Check sheet for the drawn part. Datum: minimum x, y, z corner. Units: mm. Round coordinates to 2 decimals unless told otherwise and drop trailing zeros. Write each loop counter-clockwise with the first axis right and the second up, starting at its lowest first coordinate (ties: lowest second). Pieces come first, ordered by that corner, then holes.
Item 1: Material ranges on line 1 (X direction, y = 33.5, z = 2.8); line 2 (Y direction, x = 46, z = 1.1), recorded low to high.
Item 2: Cross-section at B-B on z = 1.7. Enter the section's corners in (x, y).
Item 3: Cross-section at A-A on y = 2. Enter the section's corners in (x, z).
Item 4: Cross-section at C-C on x = 42.5. Enter the section's corners in (y, z).
Item 5: Go/stop test with flat-tipped pins: pin 1 Ø0.9 at (y, z) = (1.5, 2) entering from -X; pin 2 Ø1.5 at (y, z) = (34.5, 2) entering from +X. Record where each tip stops, or that it passes through.
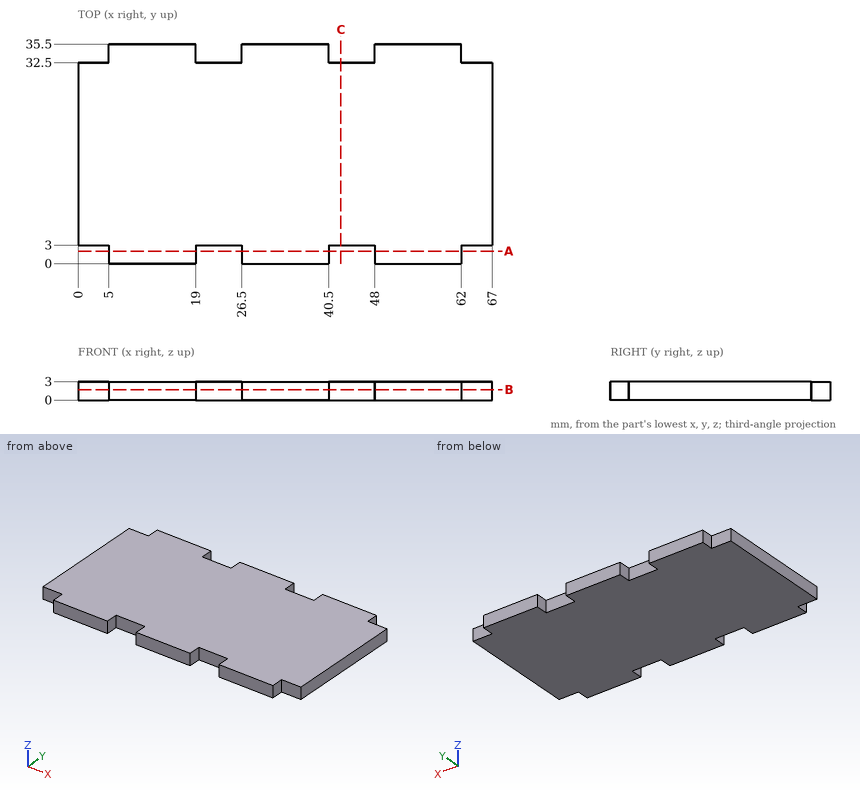
Response values:
1. line 1: x = 5 to 19, 26.5 to 40.5, 48 to 62
1. line 2: y = 3 to 32.5
2. outline: (0, 3) - (5, 3) - (5, 0) - (19, 0) - (19, 3) - (26.5, 3) - (26.5, 0) - (40.5, 0) - (40.5, 3) - (48, 3) - (48, 0) - (62, 0) - (62, 3) - (67, 3) - (67, 32.5) - (62, 32.5) - (62, 35.5) - (48, 35.5) - (48, 32.5) - (40.5, 32.5) - (40.5, 35.5) - (26.5, 35.5) - (26.5, 32.5) - (19, 32.5) - (19, 35.5) - (5, 35.5) - (5, 32.5) - (0, 32.5) - close
3. outline: (5, 0) - (19, 0) - (19, 3) - (5, 3) - close; (26.5, 0) - (40.5, 0) - (40.5, 3) - (26.5, 3) - close; (48, 0) - (62, 0) - (62, 3) - (48, 3) - close
4. outline: (3, 0) - (32.5, 0) - (32.5, 3) - (3, 3) - close
5. pin 1: stops at x = 5
5. pin 2: stops at x = 62
